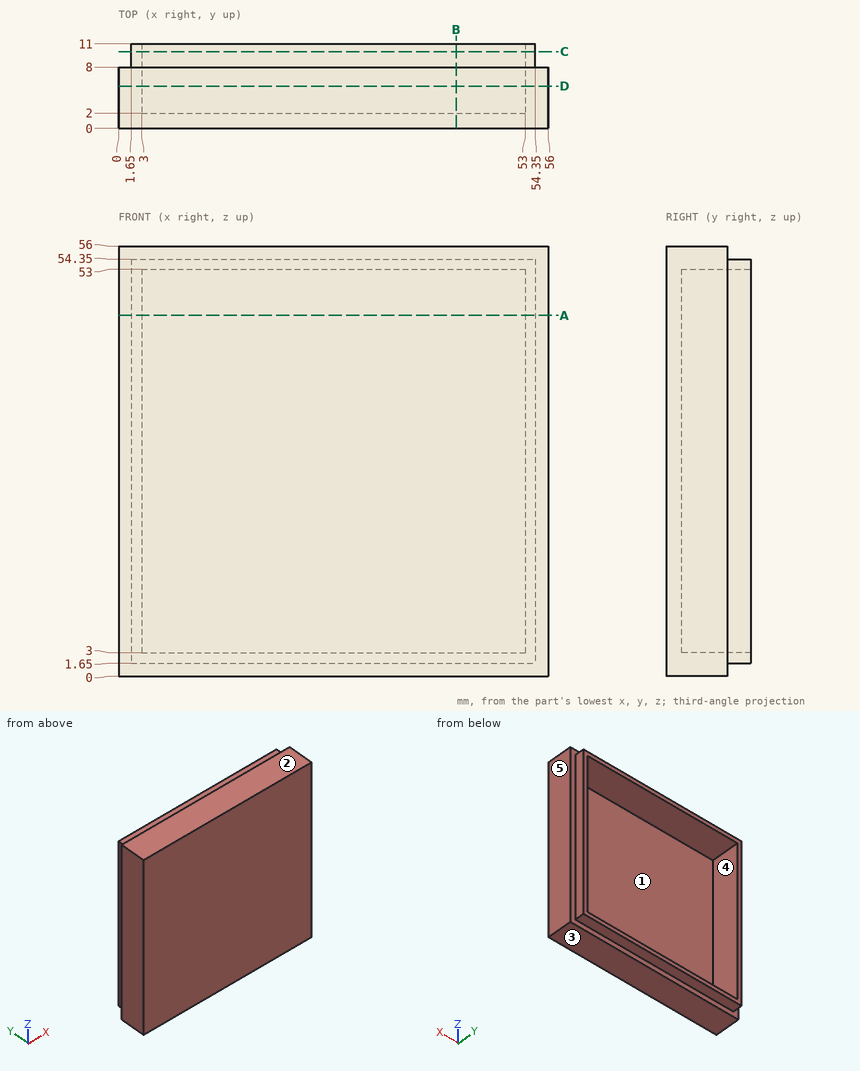
Geometry check sheet. Reference: drawing and pictorial views, mm from the part's lowest x, y, z. A direction names the side the tool comes from. Coordinates: 2 decimals unless noted, no trailing zeros. Order: outer loops, then holes, each group sorted by start corner. A loop starts at its lowest first (then second) coordinate and runs counter-clockwise, first axis right, second up.
Item 1: Section check A-A (z = 47). Enter the section's corners in (x, y).
Item 2: Section check D-D (y = 5.5). Enter the section's corners in (x, z).
Item 3: Depth check by flat-ended pin: pin 1 (5 mm diameter, centred on x = 35, z = 22.5, fed in from +Y); pin 2 (3.5 mm diameter, centred on x = 40.5, y = 10, fed in from -Z); pin 3 (1.5 mm diameter, centred on y = 10, z = 18, fed in from -X). Enter the tip coordinate at first touch or a pass-through.
Item 4: Mould release check, pull along X, two halves, no side actions. Record for the marked faces 3, 4 and 5: released by +X, released by -X, zero draft, split by the parting line, or undercut.
Item 5: Tool access check on the marked faces 1 and 2. Record the directions out of +Z, -Z, +X, -X, +Y, -Y that give a thin tool (end or side, any length) a straight path to the whole face; none if there is none.
Item 6: Scan lines: line 1 along X through (y, z) = (2.5, 42); line 2 along X through (y, z) = (9, 51). Record each from-to range of solid material in increasing order.
Item 7: Section check B-B (x = 44). Enter the section's corners in (y, z).
Item 8: Section check C-C (y = 10). Enter the section's corners in (x, z).
Check sheet entries:
1. outline: (0, 0) - (56, 0) - (56, 8) - (54.35, 8) - (54.35, 11) - (53, 11) - (53, 2) - (3, 2) - (3, 11) - (1.65, 11) - (1.65, 8) - (0, 8) - close
2. outline: (0, 0) - (56, 0) - (56, 56) - (0, 56) - close; hole (3, 3) - (53, 3) - (53, 53) - (3, 53) - close
3. pin 1: stops at y = 2
3. pin 2: stops at z = 1.65
3. pin 3: stops at x = 1.65
4. face 3: zero draft
4. face 4: undercut
4. face 5: released by +X
5. face 1: +Y
5. face 2: +Z, +X, -X, +Y, -Y
6. line 1: x = 0 to 3, 53 to 56
6. line 2: x = 1.65 to 3, 53 to 54.35
7. outline: (0, 0) - (8, 0) - (8, 1.65) - (11, 1.65) - (11, 3) - (2, 3) - (2, 53) - (11, 53) - (11, 54.35) - (8, 54.35) - (8, 56) - (0, 56) - close
8. outline: (1.65, 1.65) - (54.35, 1.65) - (54.35, 54.35) - (1.65, 54.35) - close; hole (3, 3) - (53, 3) - (53, 53) - (3, 53) - close
